Can you work these out from the model? Positions are in its coordinate system, mm. Face numbers are marked on the shaded views. A direction names the side the tool comes from. Give positions to 0.01 mm unless a question says otherwise; leave off trailing zeros. Order: outer loops, then holes, each group sorted by start corner. A loop starts at its lowest first (then second) coordinate and runs counter-clockwise, first axis right, second up. Notation, with made-up numbers: M -23.75,6 L 13.25,6 A24 ccw 13.25,43 Z; hole C -3.75,7.5 d4. An arc over 180 degrees is marked long. Use one line per item in the form item = value. Start each with the question number.
1. For the marked faces 1 and 2, which set-ups out of +Z, -Z, +X, -X, +Y, -Y let a thin tool reach every point of the face, with its end or its side?
2. Will these pins go through, and if not, where does the flat tip stop? P1, Ø10, axis at x = -3.5, y = 32.5, coming from the -Z side; P2, Ø6, axis at x = -11, z = -14.5, coming from the +Y side; P3, Ø4.5, axis at y = 1.5, z = -8, coming from the -X side.
3. I want a section at A-A, the plane z = -12.5. List the corners of the cut face in (x, y) for me, and give its area (3 significant figures).
4. I need wall thicknesses on L1, parallel to Y at x = 4.5, z = -0.5; L2, parallel to X at y = 1, z = -12; L3, parallel to Z at x = -0.5, y = 22. Which ranges of each line are inside material? Lowest first, please.
5. We'd pull the mould along Y, two halves only. Please class the marked faces 3, 4 and 5: +Y half, -Y half, draft (parallel to the pull), parting line (faces both ways), or undercut.
6. I want a section at B-B, the plane y = 21. List the corners of the cut face in (x, z) for me.
```python
from build123d import *

# Parameters (mm, degrees)
EXTRUDE_1_DEPTH     = 4
SKETCH_2_R          = 2.85
CUT_EXTRUDE_1_DEPTH = 10.000000000000002
EXTRUDE_2_DEPTH     = 45
FILLET_1_R          = 10
EXTRUDE_START       = -2
EXTRUDE_3_DEPTH     = 2
FILLET_2_R          = 10
FILLET_3_DEPTH      = 50
FILLET_START        = 44.37538
FILLET_3_2_DEPTH    = 5.62462
FILLET_3_3_DEPTH    = 4


with BuildPart() as part:
    # 草图1 → 凸台-拉伸1 (new body)
    with BuildSketch(Plane(origin=(0, 0, 0), x_dir=(1, 0, 0), z_dir=(0, 1, 0))):
        with BuildLine():
            ThreePointArc((-10, -25), (5.66e-15, -23.98979485566356), (10.000000000000009, -25))
            Line((10.000000000000002, -25.000000000000007), (9.999999999999996, 24.999999999999993))
            Line((9.999999999999996, 24.999999999999993), (-10.000000000000004, 24.999999999999993))
            Line((-10.000000000000004, 24.999999999999993), (-9.999999999999996, -25.000000000000007))
        make_face()
        with BuildLine():
            ThreePointArc((-23.00000000000064, -34.15262628157976), (5.42e-15, -27.98979485566356), (23.000000000000654, -34.15262628157976))
            Line((23.000000000000064, -34.15262628157941), (25.00000000000006, -30.688524666441673))
            ThreePointArc((25.000000000000064, -30.688524666441666), (17.729631361654985, -27.23875024936818), (10.000000000000009, -25))
            Line((10.000000000000004, -25.000000000000007), (-9.999999999999996, -25.000000000000007))
            ThreePointArc((-10, -25), (-17.72963136165498, -27.23875024936818), (-25.000000000000064, -30.688524666441673))
            Line((-25.00000000000006, -30.688524666441673), (-23.000000000000057, -34.152626281579415))
        make_face()
        with BuildLine():
            Line((-9.999999999999996, -25.000000000000007), (10.000000000000004, -25.000000000000007))
            ThreePointArc((10.000000000000009, -25), (5.66e-15, -23.98979485566356), (-10, -25))
        make_face()
    extrude(amount=EXTRUDE_1_DEPTH)

    # 草图2 → 切除-拉伸1 (cut)
    with BuildSketch(Plane(origin=(0, 4, 0), x_dir=(1, 0, 0), z_dir=(0, 1, 0))):
        with Locations(Location((-1.73e-15, 12.499999999999996, 0), (0, 0, 270))):
            Circle(SKETCH_2_R)
    extrude(amount=-CUT_EXTRUDE_1_DEPTH, mode=Mode.SUBTRACT)

    # 草图3 → 凸台-拉伸2 (add)
    with BuildSketch(Plane(origin=(0, 4, 0), x_dir=(1, 0, 0), z_dir=(0, 1, 0))):
        with BuildLine():
            ThreePointArc((9.999999999999995, -25.000000000000007), (5.66e-15, -23.989794855663575), (-9.999999999999996, -25.000000000000014))
            ThreePointArc((-9.999999999999996, -25.000000000000014), (-17.729631361654977, -27.238750249368195), (-25.000000000000057, -30.68852466644168))
            Line((-25.000000000000064, -30.68852466644167), (-23.00000000000006, -34.152626281579415))
            ThreePointArc((-23.000000000000064, -34.152626281579415), (-5.33e-15, -27.98979485566356), (23.000000000000064, -34.15262628157941))
            Line((23.000000000000057, -34.152626281579415), (25.00000000000006, -30.688524666441673))
            ThreePointArc((25.000000000000057, -30.68852466644168), (17.72963136165498, -27.238750249368195), (9.999999999999995, -25.000000000000007))
        make_face()
    extrude(amount=EXTRUDE_2_DEPTH)

    # 倒角1
    # the kernel refuses this chamfer: 25.647736894, 20 mm, written as the material it adds along each edge
    with BuildSketch(Plane(origin=(10.000000000000004, 0, 25.00000000000001), x_dir=(-2.4e-16, 0, -1), z_dir=(0, 1, 0))) as chamfer_1_piece_1_section:
        with BuildLine():
            Line((15.870240384772439, 0.6233017511174166), (-7.473452483423025, -17.23288480714665))
            Line((-7.473452483423025, -17.23288480714665), (-7.907732226484158, -16.959894573117097))
            ThreePointArc((-7.907732226484158, -16.959894573117097), (-3.2240953608677487, -8.827331157857245), (-0.5025909475750687, 0.10259094757506672))
            Line((-0.5025909475750687, 0.10259094757506672), (1.2e-16, 0.5129547378753365))
            ThreePointArc((1.2e-16, 0.5129547378753365), (7.9351201923862185, 0.5129547378753364), (15.870240384772439, 1.136256488992753))
            Line((15.870240384772439, 1.136256488992753), (15.870240384772439, 0.6233017511174166))
        make_face()
    chamfer_1_piece_1 = extrude(amount=4, mode=Mode.PRIVATE)
    chamfer_1_piece_1 = split(chamfer_1_piece_1, bisect_by=Plane(origin=(23.713203435596473, 0, 32.91732169499376), z_dir=(-0.8660254037844379, 0, -0.5000000000000014)), keep=Keep.TOP, mode=Mode.PRIVATE)
    add(chamfer_1_piece_1)
    with BuildSketch(Plane(origin=(-9.999999999999996, 0, 25.000000000000007), x_dir=(-1.2e-16, 0, -1), z_dir=(0, 1, 0))) as chamfer_1_piece_2_section:
        with BuildLine():
            Line((15.8702403847722, -0.6233017511174258), (-7.473452483423406, 17.232884807146757))
            Line((-7.473452483423406, 17.232884807146757), (-7.907732226484546, 16.959894573117197))
            ThreePointArc((-7.907732226484546, 16.959894573117197), (-3.224095360867959, 8.827331157857294), (-0.5025909475750723, -0.10259094757507187))
            Line((-0.5025909475750723, -0.10259094757507187), (-6e-17, -0.5129547378753436))
            ThreePointArc((-6e-17, -0.5129547378753436), (7.935120192386101, -0.5129547378753427), (15.8702403847722, -1.1362564889927693))
            Line((15.8702403847722, -1.1362564889927693), (15.8702403847722, -0.6233017511174258))
        make_face()
    chamfer_1_piece_2 = extrude(amount=4, mode=Mode.PRIVATE)
    chamfer_1_piece_2 = split(chamfer_1_piece_2, bisect_by=Plane(origin=(-23.713203435596462, 0, 32.917321694993774), z_dir=(0.8660254037844375, 0, -0.500000000000002)), keep=Keep.TOP, mode=Mode.PRIVATE)
    add(chamfer_1_piece_2)

    # 圆角1
    fillet_1_edges = [part.edges().sort_by_distance(p)[0] for p in [
        (3.375e-14, 4, 23.989794855663604),
    ]]
    fillet(fillet_1_edges, radius=FILLET_1_R)

    # 草图4 → 凸台-拉伸3 (add)
    with BuildSketch(Plane(origin=(0, 49, 0), x_dir=(1, 0, 0), z_dir=(0, 1, 0)).offset(EXTRUDE_START)):
        with BuildLine():
            Line((-27.00000000000007, -27.22442305130391), (-25.00000000000007, -30.68852466644167))
            ThreePointArc((-25.00000000000007, -30.68852466644167), (5.66e-15, -23.98979485566357), (25.00000000000006, -30.688524666441673))
            Line((25.00000000000006, -30.688524666441673), (27.00000000000007, -27.22442305130391))
            ThreePointArc((27.00000000000007, -27.22442305130391), (5.91e-15, -19.989794855663554), (-27.00000000000007, -27.22442305130391))
        make_face()
    extrude(amount=EXTRUDE_3_DEPTH)

    # 圆角2
    # the kernel refuses this fillet: 10 mm, written as the material it adds along each edge
    with BuildSketch(Plane(origin=(-7.11e-15, 47, 73.9897948556636), x_dir=(-0.5000000000000009, 0, -0.8660254037844382), z_dir=(-0.8660254037844382, 0, 0.5000000000000009))) as fillet_2_piece_1:
        with BuildLine():
            CenterArc((60.000000000000014, 8.000000000000028), FILLET_2_R, 180, 53.13010235415629)
            Line((50.00000000000002, 8.000000000000028), (49.80000000000001, 8.000000000000028))
            Line((49.80000000000001, 8.000000000000028), (49.80000000000004, 0))
            Line((49.80000000000004, 0), (50.000000000000036, -0.20000000000000284))
            ThreePointArc((50.000000000000036, -0.20000000000000284), (52.000000000000036, -0.20000000000000284), (53.88000000000005, -0.1600000000000037))
            Line((53.88000000000005, -0.1600000000000037), (54.00000000000006, 0))
        make_face()
    revolve(axis=Axis((-7.11e-15, 47, 73.9897948556636), (0, -1, 0)), revolution_arc=60.000000000000135)

    # 圆角3: read off the stored shape, not the designer's step
    # 圆角3 outline → 圆角3 (cut)
    with BuildSketch(Plane(origin=(0, 0, 0), x_dir=(1, 0, 0), z_dir=(0, 1, 0))):
        with BuildLine():
            ThreePointArc((-23, -34.152626282), (-23.374473484, -29.343864194), (-21.454427524, -24.919178135))
            Line((-21.454427524, -24.919178135), (-20.904466424, -24.200204744))
            ThreePointArc((-20.904466424, -24.200204744), (-23.999915623, -25.616206503), (-27, -27.224423051))
            Line((-27, -27.224423051), (-23, -34.152626282))
        make_face()
        with BuildLine():
            Line((23, -34.152626282), (27, -27.224423051))
            ThreePointArc((27, -27.224423051), (23.999915623, -25.616206503), (20.904466424, -24.200204744))
            Line((20.904466424, -24.200204744), (21.454427366, -24.919177929))
            ThreePointArc((21.454427366, -24.919177929), (23.374473462, -29.343864066), (23, -34.152626282))
        make_face()
        with BuildLine():
            Line((-10, 25), (-10, 15))
            ThreePointArc((-10, 15), (-7.071067812, 22.071067812), (0, 25))
            Line((0, 25), (-10, 25))
        make_face()
        with BuildLine():
            Line((10, 25), (0, 25))
            ThreePointArc((0, 25), (7.071067812, 22.071067812), (10, 15))
            Line((10, 15), (10, 25))
        make_face()
    extrude(amount=FILLET_3_DEPTH, mode=Mode.SUBTRACT)

    # Fillet 3 2 outline → Fillet 3 2 (cut)
    with BuildSketch(Plane(origin=(0, 0, 0), x_dir=(1, 0, 0), z_dir=(0, 1, 0)).offset(FILLET_START)):
        with BuildLine():
            Line((-20.904466424, -24.200204744), (-21.454427524, -24.919178135))
            ThreePointArc((-21.454427524, -24.919178135), (-21.143258439, -24.532645684), (-20.813297877, -24.162025174))
            ThreePointArc((-20.813297877, -24.162025174), (-20.858890886, -24.1810941), (-20.904466424, -24.200204744))
        make_face()
        with BuildLine():
            ThreePointArc((20.904466424, -24.200204744), (20.858890886, -24.1810941), (20.813297877, -24.162025174))
            ThreePointArc((20.813297877, -24.162025174), (21.143258356, -24.532645585), (21.454427366, -24.919177929))
            Line((21.454427366, -24.919177929), (20.904466424, -24.200204744))
        make_face()
    extrude(amount=FILLET_3_2_DEPTH, mode=Mode.SUBTRACT)

    # Fillet 3 3 outline → Fillet 3 3 (add)
    with BuildSketch(Plane(origin=(0, 0, 0), x_dir=(1, 0, 0), z_dir=(0, 1, 0))):
        with BuildLine():
            ThreePointArc((-10, -6.558505859), (-10.528269314, -9.765734851), (-12.057263561, -12.634107711))
            Line((-12.057263561, -12.634107711), (-10, -9.944612473))
            Line((-10, -9.944612473), (-10, -6.558505859))
        make_face()
        with BuildLine():
            Line((10, -9.944612473), (12.057263561, -12.634107711))
            ThreePointArc((12.057263561, -12.634107711), (10.528269314, -9.765734851), (10, -6.558505859))
            Line((10, -6.558505859), (10, -9.944612473))
        make_face()
    extrude(amount=FILLET_3_3_DEPTH)


solid = part.part
```
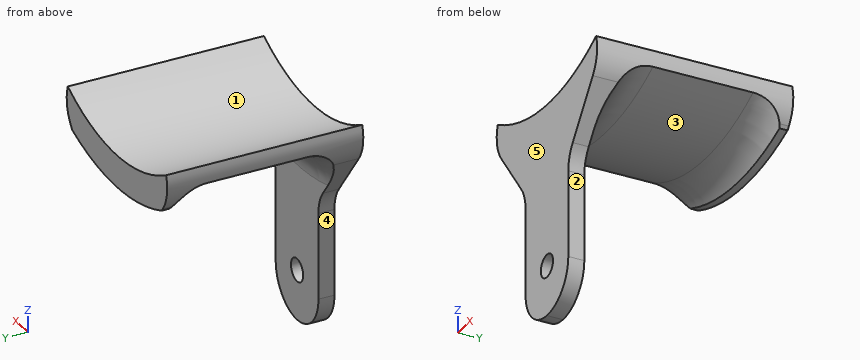
Check result:
q1.face_1 = +Z, +Y, -Y
q1.face_2 = -Z, +X, +Y, -Y
q2.P1 = 23.99
q2.P2 = 4
q2.P3 = -10
q3.outline = M -10,0 L -2.85,0 L -2.85,4 L -10,4 Z; M 2.85,0 L 10,0 L 10,4 L 2.85,4 Z
q3.area = 57.2 mm2
q4.L1 = 0 to 4
q4.L2 = -10 to -2.81, 2.81 to 10
q4.L3 = 23.99 to 27.99
q5.face_3 = undercut
q5.face_4 = draft
q5.face_5 = -Y half
q6.outline = M -23.44,29.83 A50 ccw 23.44,29.83 A10 ccw 23,34.15 A46 cw -23,34.15 A10 ccw Z
